For this review, take the finished solid that the model builds, in its own axes (mm). A direction names the side the tool comes from. Give positions to 0.01 mm unless a question says otherwise; leave off trailing zeros. Loops run counter-clockwise (first coordinate to the right, second up) from the corner with the lowest first, then second, coordinate; pieces in that order, holes last. Notation, with made-up numbers: (-11, 75.5) - (16, 75.5) arc R26 cw to (16, 109.5) - close; hole circle Ø10 at (-29.75, 26.25). An arc over 180 degrees is marked (long way). Answer in a Markdown table with one row per item.
```python
from build123d import *

# Parameters (mm, degrees)
SKETCH1_W                 = 45
SKETCH1_H                 = 21
BOSS_EXTRUDE1_DEPTH       = 20
SKETCH2_R                 = 2.75
ALIGNMENTHOLES_DEPTH      = 21
SKETCH4_R                 = 8.5
PIEZOCUT_DEPTH            = 3
F_0_535_40_TAPPED_HOLE1_D = 12.7
F_8_32_TAPPED_HOLE2_D     = 3.4544
F_8_32_TAPPED_HOLE2_DEPTH = 10
F_8_32_TAPPED_HOLE2_TIP   = 1.037806461


with BuildPart() as part:
    # Sketch1 → Boss-Extrude1 (new body)
    with BuildSketch(Plane(origin=(0, 0, 0), x_dir=(1, 0, 0), z_dir=(0, 1, 0))):
        with Locations((22.5, 10.5)):
            Rectangle(SKETCH1_W, SKETCH1_H)
    extrude(amount=BOSS_EXTRUDE1_DEPTH)

    # Sketch2 → AlignmentHoles (cut, through all)
    with BuildSketch(Plane.XZ):
        with Locations((39.5, -16.5)):
            Circle(SKETCH2_R)
        with Locations((39.5, -4.5)):
            Circle(SKETCH2_R)
        with Locations((5.5, -16.5)):
            Circle(SKETCH2_R)
        with Locations((5.5, -4.5)):
            Circle(SKETCH2_R)
    extrude(amount=-ALIGNMENTHOLES_DEPTH, mode=Mode.SUBTRACT)

    # Sketch4 → PiezoCut (cut)
    with BuildSketch(Plane(origin=(0, 20, 0), x_dir=(1, 0, 0), z_dir=(0, 1, 0))):
        with Locations((22.5, 10.5)):
            Circle(SKETCH4_R)
    extrude(amount=-PIEZOCUT_DEPTH, mode=Mode.SUBTRACT)

    # 0.535-40 Tapped Hole1 (through all)
    with Locations(Plane(origin=(0, 0, 0), x_dir=(-1, 0, 0), z_dir=(0, -1, 0))):
        with Locations((-22.5, 10.5)):
            Hole(F_0_535_40_TAPPED_HOLE1_D / 2)

    # #8-32 Tapped Hole2
    with Locations(Plane(origin=(0, 0, -21), x_dir=(-1, 0, 0), z_dir=(0, 0, -1))):
        with Locations((-22.5, 10)):
            Hole(F_8_32_TAPPED_HOLE2_D / 2, depth=F_8_32_TAPPED_HOLE2_DEPTH)
            with Locations((0, 0, -(F_8_32_TAPPED_HOLE2_DEPTH + F_8_32_TAPPED_HOLE2_TIP / 2))):  # 118° drill point
                Cone(0, F_8_32_TAPPED_HOLE2_D / 2, F_8_32_TAPPED_HOLE2_TIP, mode=Mode.SUBTRACT)


solid = part.part
```
1. We need section C-C, the plane z = -6.5. Give the boundary of the cut face in (x, y), and give its area (3 significant figures).
Values:
| item | result |
|---|---|
| outline | (0, 0) - (3.61, 0) - (3.61, 20) - (0, 20) - close; (7.39, 0) - (17.57, 0) - (17.57, 17) - (15, 17) - (15, 20) - (7.39, 20) - close; (27.43, 0) - (37.61, 0) - (37.61, 20) - (30, 20) - (30, 17) - (27.43, 17) - close; (41.39, 0) - (45, 0) - (45, 20) - (41.39, 20) - close |
| area | 536 mm^2 |
2. We need section A-A, the plane x = 39.5. Give the boundary of the cut face in (y, z).
Values:
| item | result |
|---|---|
| outline | (0, -21) - (20, -21) - (20, -19.25) - (0, -19.25) - close; (0, -13.75) - (20, -13.75) - (20, -7.25) - (0, -7.25) - close; (0, -1.75) - (20, -1.75) - (20, 0) - (0, 0) - close |
3. Mouldability with a two-part tool opening along Z and no side actions: class faces 4 (the face through (22, 10, 0)), 5 (the face through (45, 10, -10)), 6 (the face through (6.77, 9.86, -6.94)) as released by +Z, released by -Z, zero draft, split by the parting line, or undercut.
Values:
| item | result |
|---|---|
| face 4 | released by +Z |
| face 5 | zero draft |
| face 6 | undercut |
4. We need section B-B, the plane y = 10. Give the boundary of the cut face in (x, z).
Values:
| item | result |
|---|---|
| outline | (0, -21) - (20.77, -21) - (20.77, -16.61) arc R6.35 cw (long way) to (24.23, -16.61) - (24.23, -21) - (45, -21) - (45, 0) - (0, 0) - close; hole circle Ø5.5 at (5.5, -16.5); hole circle Ø5.5 at (5.5, -4.5); hole circle Ø5.5 at (39.5, -16.5); hole circle Ø5.5 at (39.5, -4.5) |
5. Wall thickness on line 1 (Z direction, x = 39.5, y = 13.5); line 2 (X direction, y = 1.5, z = -6.25); line 3 (Z direction, x = 22.5, y = 18.4): over which ranges is each line inside the solid? List them lowest first. Write a range as [from, to].
Values:
| item | result |
|---|---|
| line 1 | z = [-21, -19.25], [-13.75, -7.25], [-1.75, 0] |
| line 2 | x = [0, 3.38], [7.62, 17.78], [27.22, 37.38], [41.62, 45] |
| line 3 | z = [-21, -19], [-2, 0] |
6. We need section D-D, the plane x = 22.5. Give the boundary of the cut face in (y, z), and give its area (3 significant figures).
Values:
| item | result |
|---|---|
| outline | (0, -21) - (8.27, -21) - (8.27, -16.85) - (0, -16.85) - close; (0, -4.15) - (17, -4.15) - (17, -2) - (20, -2) - (20, 0) - (0, 0) - close; (11.73, -21) - (20, -21) - (20, -19) - (17, -19) - (17, -16.85) - (11.73, -16.85) - close |
| area | 139 mm^2 |
7. For faces 1 (the face through (24.147, 10.519, -18.771)), 2 (the face through (36.753, 9.86, -16.379)), 3 (the face through (16, 17, -10)), list the 3-axis set-ups (+Z, -Z, +X, -X, +Y, -Y) from which the entire face can be reached by the end or side of a thin tool; tool diameter is ignored.
Values:
| item | result |
|---|---|
| face 1 | -Z |
| face 2 | +Y, -Y |
| face 3 | +Y |
